The model under review builds one solid part; all positions refer to its coordinate system, in mm. A direction names the side the tool comes from. Coordinates: 2 decimals unless noted, no trailing zeros. Order: outer loops, then holes, each group sorted by start corner. A loop starts at its lowest first (then second) coordinate and runs counter-clockwise, first axis right, second up. Notation, with made-up numbers: M -22,27.5 L 17,27.5 A19 ccw 17,43.5 Z; hole C 36.25,16 d10. An arc over 180 degrees is marked long. Write each question's results on one line, items separated by ' | '.
from build123d import *

# Parameters (mm, degrees)
F0_R     = 2.1
F1_DEPTH = 6.16
F2_W     = 23
F2_H     = 3
F3_DEPTH = 14.2
F4_W     = 23
F4_H     = 20
F4_W_2   = 2.2
F4_H_2   = 1.7
F5_DEPTH = 1.6
F8_DEPTH = 2
F12_R    = 2


with BuildPart() as f1:
    # F0 (on Right) → F1 (new body)
    with BuildSketch(Plane.YZ):
        Polygon((-9.7124977037, -5.25), (9.7124977037, -5.25), (11.5, -3.4624977037), (11.5, 3.4624977037), (11.5, 5.25), (9.7124977037, 5.25), (-9.7124977037, 5.25), (-11.5, 5.25), (-11.5, 3.4624977037), (-11.5, -3.4624977037), align=None)
        with Locations((-6.35, 0)):
            Circle(F0_R, mode=Mode.SUBTRACT)
        with Locations((6.35, 0)):
            Circle(F0_R, mode=Mode.SUBTRACT)
    extrude(amount=F1_DEPTH)

    # F2 (on face) → F3 (join)
    with BuildSketch(Plane(origin=(0, 0, 0), x_dir=(0, -1, 0), z_dir=(-1, 0, 0))):
        with Locations((0, 6.75)):
            Rectangle(F2_W, F2_H)
    extrude(amount=-F3_DEPTH)

    # F4 (on face) → F5 (join)
    with BuildSketch(Plane.YZ.offset(14.2)):
        with Locations((0, 15.25)):
            Rectangle(F4_W, F4_H)
        with Locations((-2.65, 9.4)):
            Rectangle(F4_W_2, F4_H_2, mode=Mode.SUBTRACT)
        with Locations((2.65, 9.4)):
            Rectangle(F4_W_2, F4_H_2, mode=Mode.SUBTRACT)
        with Locations((-2.65, 23.1)):
            Rectangle(F4_W_2, F4_H_2, mode=Mode.SUBTRACT)
        with Locations((2.65, 23.1)):
            Rectangle(F4_W_2, F4_H_2, mode=Mode.SUBTRACT)
    extrude(amount=-F5_DEPTH)

    # F6: union 

    # F7 (on face) → F8 (join)
    with BuildSketch(Plane(origin=(0, 11.5, 0), x_dir=(-1, 0, 0), z_dir=(0, 1, 0))):
        Polygon((-6.3, 8.25), (-12.6, 14.6002341062), (-12.6, 8.25), align=None)
        Polygon((-6.16, 5.25), (-14.2, 5.25), (-6.16, -1.7691504909), align=None)
    extrude(amount=-F8_DEPTH)

    # F10: F1 across plane


with BuildPart() as f1_1:
    add(f1.part)
    add(f1.part.mirror(Plane.XZ))

    # F11: F1 across plane


with BuildPart() as f1_2:
    add(f1_1.part)
    add(f1_1.part.mirror(Plane.XZ))

    # F12
    f12_edges = [f1_2.edges().sort_by_distance(p)[0] for p in [
        (13.4, 11.5, 25.25),
        (13.4, -11.5, 25.25),
    ]]
    fillet(f12_edges, radius=F12_R)


solid = f1_2.part
1) For faces 1 (the flat face through (11, -9.5, 10)), 2 (the flat face through (13, 3, 22.25)), 3 (the flat face through (0, 0, 2)), 4 (the flat face through (8, -9.5, 3)), list the 3-axis set-ups (+Z, -Z, +X, -X, +Y, -Y) from which the entire face can be reached by the end or side of a thin tool; tool diameter is ignored.
Solutions:
face 1: +Z, -X | face 2: +X, -X | face 3: +Z, -Z, -X, +Y, -Y | face 4: -Z, +X
2) Take a section at B-B on y = 6.35. State the section outline as (x, z) points.
Solutions:
outline: M 0,-5.25 L 6.16,-5.25 L 6.16,-2.1 L 0,-2.1 Z; M 0,2.1 L 6.16,2.1 L 6.16,5.25 L 14.2,5.25 L 14.2,25.25 L 12.6,25.25 L 12.6,8.25 L 0,8.25 Z
3) For pin 1 (6 mm diameter, centred on x = 8.5, y = -6, fed in from +Z); pin 2 (0.8 mm diameter, centred on x = 13, y = -2.5, fed in from -Z), all flat-tipped, find the tip position at first contact; note any pin that passes through.
Solutions:
pin 1: z = 8.25 | pin 2: z = 5.25
4) The part is to be moulded in two halves that separate along Y. For faces 5 (the flat face through (13, -3, 8.55)), 6 (the flat face through (3.04, -10.62, -4.34)), 7 (the flat face through (13, 0, 25.25)), say which applies: pulls with the +Y half, pulls with the -Y half, needs draft (parallel to the pull), parting line crosses it, or undercut.
Solutions:
face 5: undercut | face 6: pulls with the -Y half | face 7: needs draft
5) To check wall thickness, follow line 1 along Y through (x, z) = (2, 0); line 2 along Z through (x, y) = (3.75, 6.35); line 3 along Y through (x, z) = (9.5, 4). State the ranges of each line that lie inside material, in increasing order.
Solutions:
line 1: -11.5 to -8.45, -4.25 to 4.25, 8.45 to 11.5 | line 2: -5.25 to -2.1, 2.1 to 8.25 | line 3: -11.5 to -9.5, 9.5 to 11.5
6) Take a section at D-D on y = -0.25. State the section outline as (x, z) points, plus the area to 3 significant figures.
Solutions:
outline: M 0,-5.25 L 6.16,-5.25 L 6.16,5.25 L 14.2,5.25 L 14.2,25.25 L 12.6,25.25 L 12.6,8.25 L 0,8.25 Z | area: 134 mm2
7) Take a section at A-A on x = 3.5. State the section outline as (y, z) points.
Solutions:
outline: M -11.5,-3.46 L -9.71,-5.25 L 9.71,-5.25 L 11.5,-3.46 L 11.5,8.25 L -11.5,8.25 Z; hole C -6.35,0 d4.2; hole C 6.35,0 d4.2
8) Take a section at C-C on z = 0. State the section outline as (x, y) points.
Solutions:
outline: M 0,-11.5 L 8.19,-11.5 L 8.19,-9.5 L 6.16,-9.5 L 6.16,-8.45 L 0,-8.45 Z; M 0,-4.25 L 6.16,-4.25 L 6.16,4.25 L 0,4.25 Z; M 0,8.45 L 6.16,8.45 L 6.16,9.5 L 8.19,9.5 L 8.19,11.5 L 0,11.5 Z
